Can you work these out from the model? Positions are in its coordinate system, mm. Round coordinates to 2 decimals unless told otherwise and drop trailing zeros. One line per item, written item: value. Start each with the question number.
(1) I'm going to push flat-ended pins straight in: pin 1 Ø0.9 at (y, z) = (47.5, 1.5) entering from -X; pin 2 Ø0.9 at (x, z) = (307, 1) entering from +Y. Where does each tip first touch, or does it pass through?
(2) If I drill on L1, parallel to X at y = 51.5, z = 1.15; L2, parallel to Y at x = 44.5, z = 2.3; L3, parallel to Y at x = 74, z = 2.85, over which ranges is the centre line in solid material (lowest first)? Write a range as from..to.
(3) I want a section at A-A on z = 1.5. Give the number of separate pieces and of enclosed holes in the cut face, plus the area to 3 significant figures.
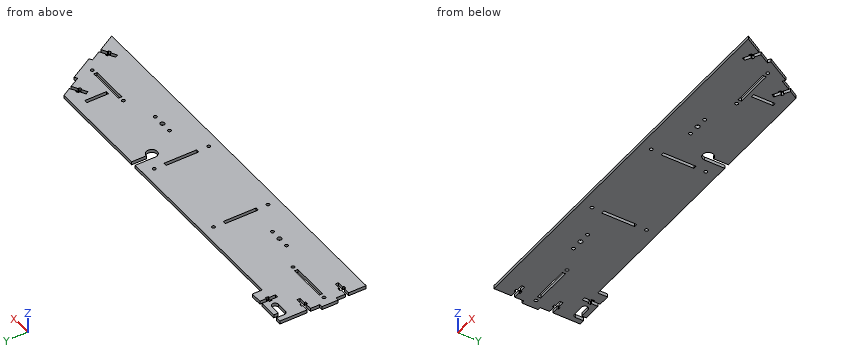
from build123d import *

# Parameters (mm, degrees)
SKETCH_1_R             = 2
SKETCH_1_R_2           = 1.5
EXTRUDE_1_DEPTH        = 3
SKETCH_2_W             = 19
SKETCH_2_H             = 3
EXTRUDE_2_DEPTH        = 3
PATTERN_LINEAR_1_COUNT = 9
PATTERN_LINEAR_1_PITCH = 28
SKETCH_3_W             = 3
SKETCH_3_H             = 30
CUT_EXTRUDE_1_DEPTH    = 3
SKETCH_4_W             = 35
SKETCH_4_H             = 3
CUT_EXTRUDE_2_DEPTH    = 3
SKETCH_5_R             = 1.5
CUT_EXTRUDE_3_DEPTH    = 3
CUT_EXTRUDE_4_DEPTH    = 3
CUT_EXTRUDE_5_DEPTH    = 3
SKETCH_8_W             = 39
SKETCH_8_H             = 3
EXTRUDE_3_DEPTH        = 9
SKETCH_11_W            = 3
SKETCH_11_H            = 25
EXTRUDE_5_DEPTH        = 3
SKETCH_12_W            = 3
SKETCH_12_H            = 15
EXTRUDE_6_DEPTH        = 3
SKETCH_13_W            = 243
SKETCH_13_H            = 3
CUT_EXTRUDE_7_DEPTH    = 3
SKETCH_14_W            = 3
SKETCH_14_H            = 20
CUT_EXTRUDE_8_DEPTH    = 10
CUT_EXTRUDE_9_DEPTH    = 3
CUT_EXTRUDE_10_DEPTH   = 10
CUT_EXTRUDE_11_DEPTH   = 10


with BuildPart() as part:
    # Эскиз1 → Бобышка-Вытянуть1 (new body)
    with BuildSketch(Plane.XY):
        Polygon((320, 70), (360.414518843, 0), (0, 0), (0, 70), align=None)
        with Locations((84, 25)):
            Circle(SKETCH_1_R, mode=Mode.SUBTRACT)
        with Locations((250, 25)):
            Circle(SKETCH_1_R, mode=Mode.SUBTRACT)
        with Locations((94, 25)):
            Circle(SKETCH_1_R_2, mode=Mode.SUBTRACT)
        with Locations((74, 25)):
            Circle(SKETCH_1_R_2, mode=Mode.SUBTRACT)
        with Locations((240, 25)):
            Circle(SKETCH_1_R_2, mode=Mode.SUBTRACT)
        with Locations((260, 25)):
            Circle(SKETCH_1_R_2, mode=Mode.SUBTRACT)
    extrude(amount=EXTRUDE_1_DEPTH)

    # Эскиз2 → Бобышка-Вытянуть2 (add)
    with BuildSketch(Plane(origin=(0, 70, 0), x_dir=(1, 0, 0), z_dir=(0, 1, 0))):
        with Locations((291.5, -1.5)):
            Rectangle(SKETCH_2_W, SKETCH_2_H)
    extrude_2 = extrude(amount=EXTRUDE_2_DEPTH)

    # Линейный массив1: Бобышка-Вытянуть2 ×9
    with Locations(*[(-i * PATTERN_LINEAR_1_PITCH, 0, 0) for i in range(1, PATTERN_LINEAR_1_COUNT)]):
        add(extrude_2)

    # Эскиз3 → Вырез-Вытянуть1 (cut)
    with BuildSketch(Plane.XY.offset(3)):
        with Locations((207.5, 35)):
            Rectangle(SKETCH_3_W, SKETCH_3_H)
        with Locations((123.5, 35)):
            Rectangle(SKETCH_3_W, SKETCH_3_H)
    extrude(amount=-CUT_EXTRUDE_1_DEPTH, mode=Mode.SUBTRACT)

    # Эскиз4 → Вырез-Вытянуть2 (cut)
    with BuildSketch(Plane.XY.offset(3)):
        with Locations((311.841234018, 35)):
            Rectangle(SKETCH_4_W, SKETCH_4_H)
        with Locations((27.5, 35)):
            Rectangle(SKETCH_4_W, SKETCH_4_H)
    extrude(amount=-CUT_EXTRUDE_2_DEPTH, mode=Mode.SUBTRACT)

    # Эскиз5 → Вырез-Вытянуть3 (cut)
    with BuildSketch(Plane.XY.offset(3)):
        with Locations((5.5, 35)):
            Circle(SKETCH_5_R)
        with Locations((49.5, 35)):
            Circle(SKETCH_5_R)
        with Locations((123.5, 60)):
            Circle(SKETCH_5_R)
        with Locations((123.5, 10)):
            Circle(SKETCH_5_R)
        with Locations((207.5, 60)):
            Circle(SKETCH_5_R)
        with Locations((207.5, 10)):
            Circle(SKETCH_5_R)
        with Locations((289.841234018, 35)):
            Circle(SKETCH_5_R)
        with Locations((333.841234018, 35)):
            Circle(SKETCH_5_R)
    extrude(amount=-CUT_EXTRUDE_3_DEPTH, mode=Mode.SUBTRACT)

    # Эскиз6 → Вырез-Вытянуть4 (cut)
    with BuildSketch(Plane.XY.offset(3)):
        Polygon((0, 54), (6, 54), (6, 55.25), (8.5, 55.25), (8.5, 54), (14.5, 54), (14.5, 51), (8.5, 51), (8.5, 49.75), (6, 49.75), (6, 51), (0, 51), align=None)
        Polygon((0, 19), (6, 19), (6, 20.25), (8.5, 20.25), (8.5, 19), (14.5, 19), (14.5, 16), (8.5, 16), (8.5, 14.75), (6, 14.75), (6, 16), (0, 16), align=None)
    extrude(amount=-CUT_EXTRUDE_4_DEPTH, mode=Mode.SUBTRACT)

    # Эскиз7 → Вырез-Вытянуть5 (cut)
    with BuildSketch(Plane.XY.offset(3)):
        Polygon((324.664518843, 61.920816371), (319.468366421, 58.920816371), (318.843366421, 60.003348125), (316.678302911, 58.753348125), (317.303302911, 57.670816371), (312.107150488, 54.670816371), (313.607150488, 52.072740159), (318.803302911, 55.072740159), (319.428302911, 53.990208405), (321.593366421, 55.240208405), (320.968366421, 56.322740159), (326.164518843, 59.322740159), align=None)
        Polygon((349.664518843, 18.619546181), (344.468366421, 15.619546181), (343.843366421, 16.702077936), (341.678302911, 15.452077936), (342.303302911, 14.369546181), (337.107150488, 11.369546181), (338.607150488, 8.77146997), (343.803302911, 11.77146997), (344.428302911, 10.688938215), (346.593366421, 11.938938215), (345.968366421, 13.02146997), (351.164518843, 16.02146997), align=None)
    extrude(amount=-CUT_EXTRUDE_5_DEPTH, mode=Mode.SUBTRACT)

    # Эскиз8 → Бобышка-Вытянуть3 (add)
    with BuildSketch(Plane(origin=(0, 70, 0), x_dir=(1, 0, 0), z_dir=(0, 1, 0))):
        with Locations((19.5, -1.5)):
            Rectangle(SKETCH_8_W, SKETCH_8_H)
    extrude(amount=EXTRUDE_3_DEPTH)

    # Эскиз11 → Бобышка-Вытянуть5 (add)
    with BuildSketch(Plane(origin=(270.310889132, 156.064064606, 0), x_dir=(0, 0, -1), z_dir=(0.8660254037844416, 0.4999999999999949, 0))):
        with Locations((-1.5, -135.207259422)):
            Rectangle(SKETCH_11_W, SKETCH_11_H)
    extrude(amount=EXTRUDE_5_DEPTH)

    # Эскиз12 → Бобышка-Вытянуть6 (add)
    with BuildSketch(Plane.ZY):
        with Locations((1.5, 35)):
            Rectangle(SKETCH_12_W, SKETCH_12_H)
    extrude(amount=EXTRUDE_6_DEPTH)

    # Эскиз13 → Вырез-Вытянуть7 (cut)
    with BuildSketch(Plane.XY.offset(3)):
        with Locations((179.5, 71.5)):
            Rectangle(SKETCH_13_W, SKETCH_13_H)
    extrude(amount=-CUT_EXTRUDE_7_DEPTH, mode=Mode.SUBTRACT)

    # Эскиз14 → Вырез-Вытянуть8 (cut)
    with BuildSketch(Plane.XY.offset(3)):
        with Locations((304.5, 50)):
            Rectangle(SKETCH_14_W, SKETCH_14_H)
    extrude(amount=-CUT_EXTRUDE_8_DEPTH, mode=Mode.SUBTRACT)

    # Эскиз15 → Вырез-Вытянуть9 (cut)
    with BuildSketch(Plane.XY.offset(3)):
        Polygon((25.5, 79), (25.5, 73), (24.25, 73), (24.25, 70.5), (25.5, 70.5), (25.5, 64.5), (28.5, 64.5), (28.5, 70.5), (29.75, 70.5), (29.75, 73), (28.5, 73), (28.5, 79), align=None)
    extrude(amount=-CUT_EXTRUDE_9_DEPTH, mode=Mode.SUBTRACT)

    # Эскиз16 → Вырез-Вытянуть10 (cut)
    with BuildSketch(Plane.XY.offset(3)):
        with BuildLine():
            Line((8.75, 74.898901738), (17.75, 74.898901738))
            ThreePointArc((17.75, 74.898901738), (20.75, 71.898901738), (17.75, 68.898901738))
            Line((17.75, 68.898901738), (7.75, 68.898901738))
            ThreePointArc((7.75, 68.898901738), (5.628679656, 69.777581394), (4.75, 71.898901738))
            Line((4.75, 71.898901738), (4.75, 79))
            Line((4.75, 79), (8.75, 79))
            Line((8.75, 79), (8.75, 74.898901738))
        make_face()
    extrude(amount=-CUT_EXTRUDE_10_DEPTH, mode=Mode.SUBTRACT)

    # Эскиз17 → Вырез-Вытянуть11 (cut)
    with BuildSketch(Plane.XY.offset(3)):
        with BuildLine():
            Line((219, 51.5), (219, 70))
            Line((219, 70), (224, 70))
            Line((224, 70), (224, 56.5))
            ThreePointArc((224, 56.5), (227.535533906, 47.964466094), (219, 51.5))
        make_face()
    extrude(amount=-CUT_EXTRUDE_11_DEPTH, mode=Mode.SUBTRACT)


solid = part.part
Established:
1. pin 1: x = 0
1. pin 2: y = 70
2. L1: 14.5..219, 229..303, 306..330.68
2. L2: 0..33.5, 36.5..70
2. L3: 0..23.5, 26.5..70
3. separate pieces: 1
3. enclosed holes: 19
3. area: 23,200 mm2
